The model under review builds one solid part; all positions refer to its coordinate system, in mm. A direction names the side the tool comes from. Coordinates: 2 decimals unless noted, no trailing zeros. Loops run counter-clockwise (first coordinate to the right, second up) from the corner with the lowest first, then second, coordinate; pieces in that order, holes last. Notation, with made-up numbers: (-7, -13) - (40, -13) arc R13 ccw to (40, -8) - close; hole circle Ø6 at (77.5, -31.75). An arc over 180 degrees is marked (long way). Use a Markdown table: item, result. Add a question column.
1) Add section D-D, the plane y = 2.9. Give the boundary of the cut face in (x, z).
2) Add section B-B, the plane x = 5. Give the boundary of the cut face in (y, z).
3) Add section C-C, the plane z = 5.5. Give the boundary of the cut face in (x, y).
4) Add section A-A, the plane y = 0.8. Give the boundary of the cut face in (x, z).
5) To check wall thickness, follow L1, parallel to X at y = 0.65, z = -5.25; L2, parallel to Z at x = 4.5, y = 1.1; L3, parallel to Y at x = 6.25, z = 0. State the ranges of each line that lie inside material, in increasing order. Write a range as [from, to].
6) Clearance check with a flat-ended pin moving along its axis: pin 1 (3 mm diameter, centred on x = 5, z = -0.5, fed in from -Y). State where the tip first meets the part, or that it passes through.
7) The part is to be moulded in two halves that separate along Z. For faces 3 (the flat face through (5, 1, 7.9)), 4 (the flat face through (8.582, 1, 0)), 5 (the flat face through (7.382, 1, 0)), 6 (the flat face through (1.882, 1, 0)), say which applies: pulls with the +Z half, pulls with the -Z half, needs draft (parallel to the pull), parting line crosses it, or undercut.
8) For faces 1 (the flat face through (5, 2, 0)), 2 (the flat face through (1, 0, 0)), list the 3-axis set-ups (+Z, -Z, +X, -X, +Y, -Y) from which the entire face can be reached by the end or side of a thin tool; tool diameter is ignored.
```python
from build123d import *

# Parameters (mm, degrees)
MAINBASESKETCH_W      = 7.9
MAINBASESKETCH_H      = 3.2
MAINBASEEXTRUDE_DEPTH = 7.9
MAINBASESHELL_T       = -1.2
CHAMFER1_SIZE         = 1.5


with BuildPart() as part:
    # MainBaseSketch → MainBaseExtrude (new, symmetric)
    with BuildSketch(Plane.XY):
        with Locations((4.631967213, 1.6)):
            Rectangle(MAINBASESKETCH_W, MAINBASESKETCH_H)
    extrude(amount=MAINBASEEXTRUDE_DEPTH, both=True)

    # MainBaseShell
    mainbaseshell_openings = [part.faces().sort_by_distance(p)[0] for p in [
        (4.631967213, 0, 0),
    ]]
    offset(amount=MAINBASESHELL_T, openings=mainbaseshell_openings, kind=Kind.INTERSECTION)

    # Chamfer1
    chamfer1_edges = [part.edges().sort_by_distance(p)[0] for p in [
        (4.631967213, 3.2, 7.9),
        (4.631967213, 3.2, -7.9),
        (0.681967213, 3.2, 0),
        (8.581967213, 3.2, 0),
    ]]
    chamfer(chamfer1_edges, length=CHAMFER1_SIZE)


solid = part.part
```
From the geometry:
| question | item | result |
|---|---|---|
| 1 | outline | (1.88, -6.7) - (7.38, -6.7) - (7.38, 6.7) - (1.88, 6.7) - close |
| 2 | outline | (0, -7.9) - (1.7, -7.9) - (3.2, -6.4) - (3.2, 6.4) - (1.7, 7.9) - (0, 7.9) - (0, 6.7) - (2, 6.7) - (2, -6.7) - (0, -6.7) - close |
| 3 | outline | (0.68, 0) - (1.88, 0) - (1.88, 2) - (7.38, 2) - (7.38, 0) - (8.58, 0) - (8.58, 1.7) - (7.08, 3.2) - (2.18, 3.2) - (0.68, 1.7) - close |
| 4 | outline | (0.68, -7.9) - (8.58, -7.9) - (8.58, 7.9) - (0.68, 7.9) - close; hole (1.88, -6.7) - (7.38, -6.7) - (7.38, 6.7) - (1.88, 6.7) - close |
| 5 | L1 | x = [0.68, 1.88], [7.38, 8.58] |
| 5 | L2 | z = [-7.9, -6.7], [6.7, 7.9] |
| 5 | L3 | y = [2, 3.2] |
| 6 | pin 1 | stops at y = 2 |
| 7 | face 3 | pulls with the +Z half |
| 7 | face 4 | needs draft |
| 7 | face 5 | undercut |
| 7 | face 6 | undercut |
| 8 | face 1 | -Y |
| 8 | face 2 | +Z, -Z, +X, -X, -Y |
